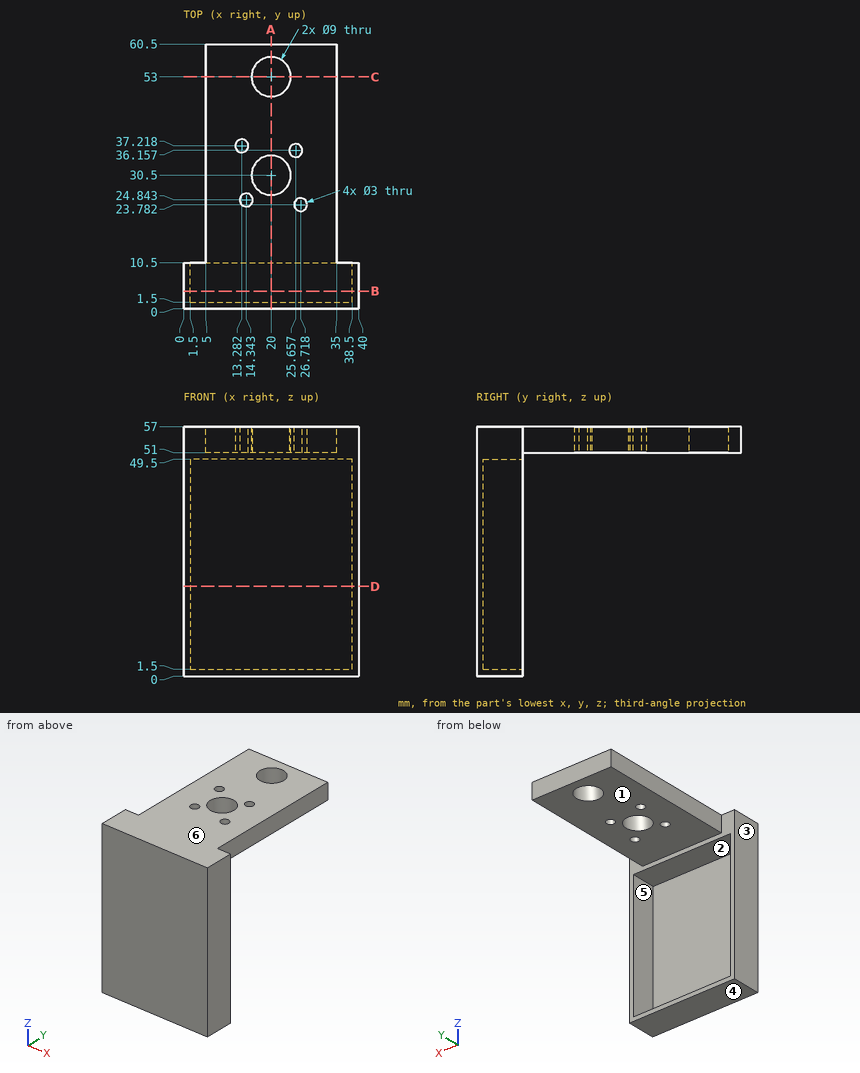
Part print with two shaded views. Sizes in mm from the minimum x, y, z corner. A direction names the side the tool comes from. Give positions to 0.01 mm unless a question says otherwise; leave off trailing zeros. Write each loop counter-clockwise with the first axis right and the second up, starting at its lowest first coordinate (ties: lowest second). Pieces come first, ordered by that corner, then holes.
1) Cut at B-B on y = 4. Write the cut outline in (x, z).
Resolved:
outline: (0, 0) - (40, 0) - (40, 57) - (0, 57) - close; hole (1.5, 1.5) - (38.5, 1.5) - (38.5, 49.5) - (1.5, 49.5) - close
2) Cut at A-A on x = 20. Write the cut outline in (y, z).
Resolved:
outline: (0, 0) - (10.5, 0) - (10.5, 1.5) - (1.5, 1.5) - (1.5, 49.5) - (10.5, 49.5) - (10.5, 51) - (26, 51) - (26, 57) - (0, 57) - close; (35, 51) - (48.5, 51) - (48.5, 57) - (35, 57) - close; (57.5, 51) - (60.5, 51) - (60.5, 57) - (57.5, 57) - close
3) Cut at C-C on y = 53. Write the cut outline in (x, z).
Resolved:
outline: (5, 51) - (15.5, 51) - (15.5, 57) - (5, 57) - close; (24.5, 51) - (35, 51) - (35, 57) - (24.5, 57) - close
4) Two-plate mould, pull along Z, no slides. Class the marked faces 4, 5 and 6: released by +Z, released by -Z, zero draft, split by the parting line, or undercut.
Resolved:
face 4: released by -Z
face 5: undercut
face 6: released by +Z
5) Probe L1, parallel to Z at x = 7.5, y = 4; L2, parallel to Y at x = 16.5, z = 54.5 (1 decimal); L3, parallel to Y at x = 30.5, z = 32. List the from-to ranges inside material, lowest first.
Resolved:
L1: z = 0 to 1.5, 49.5 to 57
L2: y = 0 to 27.7, 33.3 to 50.2, 55.8 to 60.5
L3: y = 0 to 1.5
6) Pin check, flat tips, straight feed: pin 1 (3.5 mm diameter, centred on x = 14.34, y = 24.84, fed in from -Z); pin 2 (3 mm diameter, centred on y = 41, z = 52.5, fed in from -X); pin 3 (11 mm diameter, centred on x = 25, z = 32.5, fed in from +Y); pin 4 (4.5 mm diameter, centred on x = 13.5, y = 7, fed in from -Z). Stop position of each tip, or through.
Resolved:
pin 1: stops at z = 51
pin 2: stops at x = 5
pin 3: stops at y = 1.5
pin 4: stops at z = 0
7) Cut at D-D on z = 20.5. Write the cut outline in (x, y).
Resolved:
outline: (0, 0) - (40, 0) - (40, 10.5) - (38.5, 10.5) - (38.5, 1.5) - (1.5, 1.5) - (1.5, 10.5) - (0, 10.5) - close
8) Which spindle directions (+Z, -Z, +X, -X, +Y, -Y) get a long thin tool onto all of the face, cutting with end or side? Do the marked faces 1, 2 and 3. Say none if no direction does.
Resolved:
face 1: -Z, +X, -X, +Y
face 2: +Y
face 3: +Z, -Z, -X, +Y, -Y
